from build123d import *

# Parameters (mm, degrees)
CORTAR_EXTRUIR1_DEPTH = 4.35


with BuildPart() as part:
    # Croquis1 → Revolución1 (revolve)
    with BuildSketch(Plane(origin=(0, 0, 0), x_dir=(0, 1, 0), z_dir=(0, 0, 1)), mode=Mode.PRIVATE) as revoluci_n1_sk:
        Polygon((4.025, 6.15), (4.025, 0), (8, 0), (8, 1.8), (6, 1.8), (6, 6.15), align=None)
    revolve(revoluci_n1_sk.sketch.rotate(Axis((0, 0, 0), (-1, 0, 0)), 90), axis=Axis((0, 0, 0), (-1, 0, 0)))

    # Croquis2 → Cortar-Extruir1 (cut)
    with BuildSketch(Plane(origin=(-6.15, 0, 0), x_dir=(0, -1, 0), z_dir=(-1, 0, 0))):
        with BuildLine():
            Line((-4.975, 3.354008795), (-4.975, -3.354008795))
            ThreePointArc((-4.975, -3.354008795), (-6, 0), (-4.975, 3.354008795))
        make_face()
        with BuildLine():
            Line((4.975, 3.354008795), (4.975, -3.354008795))
            ThreePointArc((4.975, -3.354008795), (6, 0), (4.975, 3.354008795))
        make_face()
    extrude(amount=-CORTAR_EXTRUIR1_DEPTH, mode=Mode.SUBTRACT)


solid = part.part
Source: CAD feature listing. Evaluate the final solid. Frame: model axes, mm. A direction names the side the tool comes from. Give positions to 0.01 mm unless a question says otherwise; leave off trailing zeros. Write each loop counter-clockwise with the first axis right and the second up, starting at its lowest first coordinate (ties: lowest second). Pieces come first, ordered by that corner, then holes. Notation, with made-up numbers: (6.25, 64) -> (27.25, 64) arc R9 cw to (27.25, 71) -> close; hole circle Ø5 at (52, -17.75). An arc over 180 degrees is marked (long way). Write item = value, one per line.
Q1. Cut plane D-D on y = -4.5. Return loops of the section in (x, z), then the cut area to 3 significant figures.
Here are the results:
outline = (-6.15, -3.97) -> (-1.8, -3.97) -> (-1.8, -6.61) -> (0, -6.61) -> (0, 6.61) -> (-1.8, 6.61) -> (-1.8, 3.97) -> (-6.15, 3.97) -> close
area = 58.3 mm²
Q2. Cut plane C-C on z = 0. Return loops of the section in (x, y) (3 decimals), then the cut area to 3 significant figures.
Here are the results:
outline = (-6.15, -4.975) -> (-1.8, -4.975) -> (-1.8, -8) -> (0, -8) -> (0, -4.025) -> (-6.15, -4.025) -> close; (-6.15, 4.025) -> (0, 4.025) -> (0, 8) -> (-1.8, 8) -> (-1.8, 4.975) -> (-6.15, 4.975) -> close
area = 22.6 mm²
Q3. Mould query, pull axis Y, two halves, no side actions, for faces 1 (the face through (-3.03, -1.21, -3.84)), 2 (the face through (-1.8, 5.2, 0.1)), 3 (the face through (-4, -4.975, 0)), 4 (the face through (-0.91, 7.81, 1.73)). Classes: +Y half, -Y half, draft (parallel to the pull), parting line (faces both ways), or undercut.
Here are the results:
face_1 = undercut
face_2 = draft
face_3 = -Y half
face_4 = parting line
Q4. First-contact query: pin 1 (7 mm diameter, centred on y = 0, z = 0, fed in from -X); pin 2 (2 mm diameter, centred on x = -1.5, y = -2, fed in from -Z); pin 3 (3 mm diameter, centred on y = -5, z = -6, fed in from -X); pin 4 (3.5 mm diameter, centred on x = -4.5, z = -0.5, fed in from -Y) (3 decimals). Flat tips, straight axial feed; report the tip coordinate or a pass-through.
Here are the results:
pin_1 = through
pin_2 = -7.94
pin_3 = -1.8
pin_4 = -4.975
Q5. Line query: line 1 (Y direction, x = -3.5, z = 0) (3 decimals); line 2 (Z direction, x = -2.75, y = 1); line 3 (Y direction, x = -1.75, z = 0.5). Output: solid intervals per line, ascending. Write a range as from..to.
Here are the results:
line_1 = -4.975..-4.025, 4.025..4.975
line_2 = -5.92..-3.9, 3.9..5.92
line_3 = -7.98..-3.99, 3.99..7.98
Q6. Reachability of faces 5 (the face through (-4, 4.975, 0)), 6 (the face through (-6.15, 1, 4.1)), 7 (the face through (-4, 0, 6)), 8 (the face through (-4, 0, -6)) from +Z, -Z, +X, -X, +Y, -Y: full face, straight path, thin tool, end or side. Return the list, or none.
Here are the results:
face_5 = +Z, -Z, -X, +Y
face_6 = +Z, -Z, -X, +Y, -Y
face_7 = +Z, -X
face_8 = -Z, -X
Q7. Cut plane B-B on x = -5. Return loops of the section in (y, z) (3 decimals).
Here are the results:
outline = (-4.975, -3.354) arc R6 ccw to (4.975, -3.354) -> (4.975, 3.354) arc R6 ccw to (-4.975, 3.354) -> close; hole circle Ø8.05 at (0, 0)
Q8. Cut plane A-A on y = 0. Return loops of the section in (x, z) (3 decimals).
Here are the results:
outline = (-6.15, -6) -> (-1.8, -6) -> (-1.8, -8) -> (0, -8) -> (0, -4.025) -> (-6.15, -4.025) -> close; (-6.15, 4.025) -> (0, 4.025) -> (0, 8) -> (-1.8, 8) -> (-1.8, 6) -> (-6.15, 6) -> close
